```python
from build123d import *
from build123d.topology import SkipClean

# Parameters (mm, degrees)
SKETCH1_R           = 6.3
SKETCH1_R_2         = 3.35
SKETCH1_R_3         = 3.1
BOSS_EXTRUDE1_DEPTH = 2.86
BOSS_EXTRUDE2_START = 1.01
SKETCH2_R           = 4.1
SKETCH2_R_2         = 3.1
BOSS_EXTRUDE2_DEPTH = 1.01
CUT_EXTRUDE1_DEPTH  = 2.76
CIRPATTERN1_COUNT   = 4


with BuildPart() as part:
    # Sketch1 → Boss-Extrude1 (new body)
    # profile 1 of 6: a face of its own
    with BuildSketch(Plane.XY):
        Circle(SKETCH1_R)
        Circle(SKETCH1_R_2, mode=Mode.SUBTRACT)
    # profile 2 of 6: a face of its own
    with BuildSketch(Plane.XY):
        Circle(SKETCH1_R_2)
        Circle(SKETCH1_R_3, mode=Mode.SUBTRACT)
    # profile 3 of 6: a face of its own
    with BuildSketch(Plane.XY):
        with BuildLine():
            ThreePointArc((3.07408523, 0.4), (2.192031022, 2.192031022), (0.4, 3.07408523))
            Line((0.4, 3.07408523), (0.4, 2.264950331))
            ThreePointArc((0.4, 2.264950331), (0.654218524, 2.204993905), (0.9, 2.116601049))
            Line((0.9, 2.116601049), (0.9, 1.05))
            ThreePointArc((0.9, 1.05), (0.943933983, 0.943933983), (1.05, 0.9))
            Line((1.05, 0.9), (2.116601049, 0.9))
            ThreePointArc((2.116601049, 0.9), (2.204993905, 0.654218524), (2.264950331, 0.4))
            Line((2.264950331, 0.4), (3.07408523, 0.4))
        make_face()
    # profile 4 of 6: a face of its own
    with BuildSketch(Plane.XY):
        with BuildLine():
            Line((0.4, -2.264950331), (0.4, -3.07408523))
            ThreePointArc((0.4, -3.07408523), (2.192031022, -2.192031022), (3.07408523, -0.4))
            Line((3.07408523, -0.4), (2.264950331, -0.4))
            ThreePointArc((2.264950331, -0.4), (2.204993905, -0.654218524), (2.116601049, -0.9))
            Line((2.116601049, -0.9), (1.05, -0.9))
            ThreePointArc((1.05, -0.9), (0.943933983, -0.943933983), (0.9, -1.05))
            Line((0.9, -1.05), (0.9, -2.116601049))
            ThreePointArc((0.9, -2.116601049), (0.654218524, -2.204993905), (0.4, -2.264950331))
        make_face()
    # profile 5 of 6: a face of its own
    with BuildSketch(Plane.XY):
        with BuildLine():
            Line((-1.05, -0.9), (-2.116601049, -0.9))
            ThreePointArc((-2.116601049, -0.9), (-2.204993905, -0.654218524), (-2.264950331, -0.4))
            Line((-2.264950331, -0.4), (-3.07408523, -0.4))
            ThreePointArc((-3.07408523, -0.4), (-2.192031022, -2.192031022), (-0.4, -3.07408523))
            Line((-0.4, -3.07408523), (-0.4, -2.264950331))
            ThreePointArc((-0.4, -2.264950331), (-0.654218524, -2.204993905), (-0.9, -2.116601049))
            Line((-0.9, -2.116601049), (-0.9, -1.05))
            ThreePointArc((-0.9, -1.05), (-0.943933983, -0.943933983), (-1.05, -0.9))
        make_face()
    # profile 6 of 6: a face of its own
    with BuildSketch(Plane.XY):
        with BuildLine():
            ThreePointArc((-0.4, 3.07408523), (-2.192031022, 2.192031022), (-3.07408523, 0.4))
            Line((-3.07408523, 0.4), (-2.264950331, 0.4))
            ThreePointArc((-2.264950331, 0.4), (-2.204993905, 0.654218524), (-2.116601049, 0.9))
            Line((-2.116601049, 0.9), (-1.05, 0.9))
            ThreePointArc((-1.05, 0.9), (-0.943933983, 0.943933983), (-0.9, 1.05))
            Line((-0.9, 1.05), (-0.9, 2.116601049))
            ThreePointArc((-0.9, 2.116601049), (-0.654218524, 2.204993905), (-0.4, 2.264950331))
            Line((-0.4, 2.264950331), (-0.4, 3.07408523))
        make_face()
    extrude(amount=BOSS_EXTRUDE1_DEPTH)

    # Sketch2 → Boss-Extrude2 (add)
    with SkipClean():  # the faces are left unmerged after this step: merging them gives an invalid solid
        with BuildSketch(Plane(origin=(0, 0, 0), x_dir=(-1, 0, 0), z_dir=(0, 0, -1)).offset(BOSS_EXTRUDE2_START)):
            with Locations(Location((0, 0, 0), (0, 0, 180))):
                Circle(SKETCH2_R)
            Circle(SKETCH2_R_2, mode=Mode.SUBTRACT)
        extrude(amount=-BOSS_EXTRUDE2_DEPTH)
    add(part.part.scale(1), mode=Mode.REPLACE)  # the faces are merged on a copy

    # Sketch3 → Cut-Extrude1 (cut)
    with BuildSketch(Plane.XY.offset(2.86)):
        with BuildLine():
            ThreePointArc((-1.687138839, 3.516185794), (-1.109327063, 3.738902709), (-0.503547315, 3.867355699))
            Line((-0.503547315, 3.867355699), (-0.665525593, 6.373986248))
            Line((-0.665525593, 6.373986248), (-2.918454148, 5.705545582))
            Line((-2.918454148, 5.705545582), (-1.687138839, 3.516185794))
        make_face()
        with BuildLine():
            Line((1.298290287, -2.004404983), (3.861197015, -5.383647241))
            Line((3.861197015, -5.383647241), (5.075598647, -3.732063554))
            Line((5.075598647, -3.732063554), (2.012879929, -1.304861101))
            ThreePointArc((2.012879929, -1.304861101), (1.347288977, -1.339706092), (1.298290287, -2.004404983))
        make_face()
        with BuildLine():
            ThreePointArc((-3.867355699, 0.503547315), (-3.738902709, 1.109327063), (-3.516185794, 1.687138839))
            Line((-3.516185794, 1.687138839), (-5.705545582, 2.918454148))
            Line((-5.705545582, 2.918454148), (-6.373986248, 0.665525593))
            Line((-6.373986248, 0.665525593), (-3.867355699, 0.503547315))
        make_face()
    cut_extrude1 = extrude(amount=-CUT_EXTRUDE1_DEPTH, mode=Mode.SUBTRACT)

    # CirPattern1: Cut-Extrude1 ×4 about axis
    cirpattern1_axis = Axis((0, 0, 0), (0, 0, 1))
    for i in range(1, CIRPATTERN1_COUNT):
        add(cut_extrude1.rotate(cirpattern1_axis, i * 360 / CIRPATTERN1_COUNT), mode=Mode.SUBTRACT)

    # Sketch5 → Cut-Revolve1 (revolve, cut)
    with BuildSketch(Plane(origin=(0, 0, 0), x_dir=(1, 0, 0), z_dir=(0, 1, 0)), mode=Mode.PRIVATE) as cut_revolve1_sk:
        Polygon((-6.59, -3.11), (-6.59, -1.47), (-4.85, -3.11), align=None)
    revolve(cut_revolve1_sk.sketch.rotate(Axis((0, 0, -2.797897232), (0, 0, 1)), 354.000135139), axis=Axis((0, 0, -2.797897232), (0, 0, 1)), mode=Mode.SUBTRACT)


solid = part.part
```
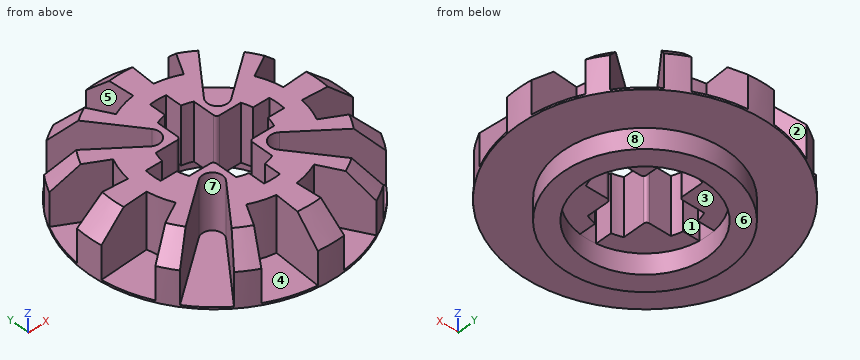
Geometry: final body of the model. Coordinates: model frame, mm. Face numbers are marked on the shaded views. A direction names the side the tool comes from. Coordinates: 2 decimals unless noted, no trailing zeros. Order: outer loops, then holes, each group sorted by start corner. A loop starts at its lowest first (then second) coordinate and runs counter-clockwise, first axis right, second up. Notation, with made-up numbers: M 58,5 L 62,5 A17 cw 62,31 Z; hole C -3.75,78.5 d8. An arc over 180 degrees is marked long. Answer in a Markdown table with one row per item. Add a question column.
Q1. Mould query, pull axis X, two halves, no side actions, for the marked faces 5, 6, 7 and 8. Classes: released by +X, released by -X, zero draft, split by the parting line, or undercut.
Q2. Section query A-A on y = 0. Return the cut outline in (x, z), and give its area (3 significant figures).
Q3. Line query: L1, parallel to Y at x = 0, z = -0.7; L2, parallel to X at y = -1.5, z = 1; L3, parallel to X at y = -4, z = 2.7. Output: solid intervals per line, ascending.
Q4. Section query C-C on z = -0.7. Return the cut outline in (x, y).
Q5. Reachability of the marked faces 1, 2, 3 and 4 from +Z, -Z, +X, -X, +Y, -Y: full face, straight path, thin tool, end or side. Return the list, or none.
Q6. Contact query for flat-ended pins moving along their axis: P1, Ø0.9, axis at y = -2, z = 1, coming from the +X side; P2, Ø1.2, axis at x = 5, y = -1.5, coming from the +Z side; P3, Ø1, axis at x = 5, z = 1.5, coming from the -Y side. Output: stop coordinate, or through.
Completed:
| question | item | result |
|---|---|---|
| 1 | face 5 | undercut |
| 1 | face 6 | zero draft |
| 1 | face 7 | undercut |
| 1 | face 8 | split by the parting line |
| 2 | outline | M -6.3,0 L -4.1,0 L -4.1,-1.01 L -3.1,-1.01 L -3.1,2.86 L -5.12,2.86 L -6.3,1.74 Z; M 3.1,-1.01 L 4.1,-1.01 L 4.1,0 L 6.3,0 L 6.3,1.74 L 5.12,2.86 L 3.1,2.86 Z |
| 2 | area | 19.0 mm2 |
| 3 | L1 | y = -4.1 to -3.1, 3.1 to 4.1 |
| 3 | L2 | x = -3.6 to -2.27, -1.24 to -0.9, 0.9 to 1.24, 2.26 to 3.6 |
| 3 | L3 | x = -2.88 to -1.96, -0.51 to 0.51, 1.96 to 2.81 |
| 4 | outline | C 0,0 d8.2; hole C 0,0 d6.2 |
| 5 | face 1 | +Z, -Z |
| 5 | face 2 | +Z, +Y |
| 5 | face 3 | -Z |
| 5 | face 4 | +Z |
| 6 | P1 | stops at x = 4.87 |
| 6 | P2 | stops at z = 0.1 |
| 6 | P3 | stops at y = -3.73 |
